The listing builds one solid part. Answer for the finished solid, in the listing's coordinates (mm). A direction names the side the tool comes from. Round coordinates to 2 decimals unless told otherwise and drop trailing zeros. Write each loop counter-clockwise with the first axis right and the second up, starting at its lowest first coordinate (ties: lowest second). Pieces come first, ordered by that corner, then holes. Notation, with made-up numbers: M 4,75.5 L 41,75.5 A13 ccw 41,85.5 Z; hole C -32.5,8 d7. An arc over 180 degrees is marked long. One line per item, written item: value. Start each with the question number.
(1) Section A-A (x = -1.75) is taken. Determine the outline of the cut face in (y, z) (1 decimal), plus the area to 3 significant figures.
(2) Section D-D (x = 1.25) is taken. Determine the outline of the cut face in (y, z) (1 decimal), plus the area to 3 significant figures.
(3) Section B-B (y = 6) is taken. Determine the outline of the cut face in (x, z).
(4) Consider probe 1 along Z at (x, y) = (4.75, 4); probe 2 along Y at (x, z) = (-2, 8); probe 3 along Y at (x, z) = (2.5, 21). Determine where each line is inside the solid, lowest interval first.
(5) Given P1, Ø5, axis at x = -4, z = 5, coming from the +Y side; P2, Ø4, axis at x = -4.5, y = -4.5, coming from the +Z side; P3, Ø2, axis at x = -3.5, z = 20, coming from the -Y side, each flat-ended and moving along its own axis, determine where each tip first touches the part or whether it passes through.
(6) For faces 1 (the flat face through (0, -8, 28.575)), 2 (the cylindrical face through (-0.688, -11.037, 14.087)), determine the directions among +Z, -Z, +X, -X, +Y, -Y from which every point of the face is accessible in a straight line to the end or side of a thin tool.
```python
from build123d import *

# Parameters (mm, degrees)
F1_DEPTH = 1.5875
F2_R     = 3.175
F3_DEPTH = 28.575


with BuildPart() as f1:
    # F0 (on Top) → F1 (new body)
    with BuildSketch(Plane.XY):
        Polygon((-8.382, -10.31875), (8.382, -15.875), (8.382, 10.31875), (-8.382, 15.875), align=None)
    extrude(amount=-F1_DEPTH)

    # F2 (on Top) → F3 (join)
    with BuildSketch(Plane.XY):
        with Locations((0, -7.9375)):
            Circle(F2_R)
    extrude(amount=F3_DEPTH)


solid = f1.part
```
Recorded:
1. outline: M -12.5,-1.6 L 13.7,-1.6 L 13.7,0 L -5.3,0 L -5.3,28.6 L -10.6,28.6 L -10.6,0 L -12.5,0 Z
1. area: 193 mm2
2. outline: M -13.5,-1.6 L 12.7,-1.6 L 12.7,0 L -5,0 L -5,28.6 L -10.9,28.6 L -10.9,0 L -13.5,0 Z
2. area: 208 mm2
3. outline: M -8.38,-1.59 L 8.38,-1.59 L 8.38,0 L -8.38,0 Z
4. probe 1: z = -1.59 to 0
4. probe 2: y = -10.4 to -5.47
4. probe 3: y = -9.89 to -5.98
5. P1: stops at y = -5.14
5. P2: stops at z = 0
5. P3: stops at y = -9.89
6. face 1: +Z, +X, -X, +Y, -Y
6. face 2: +Z
